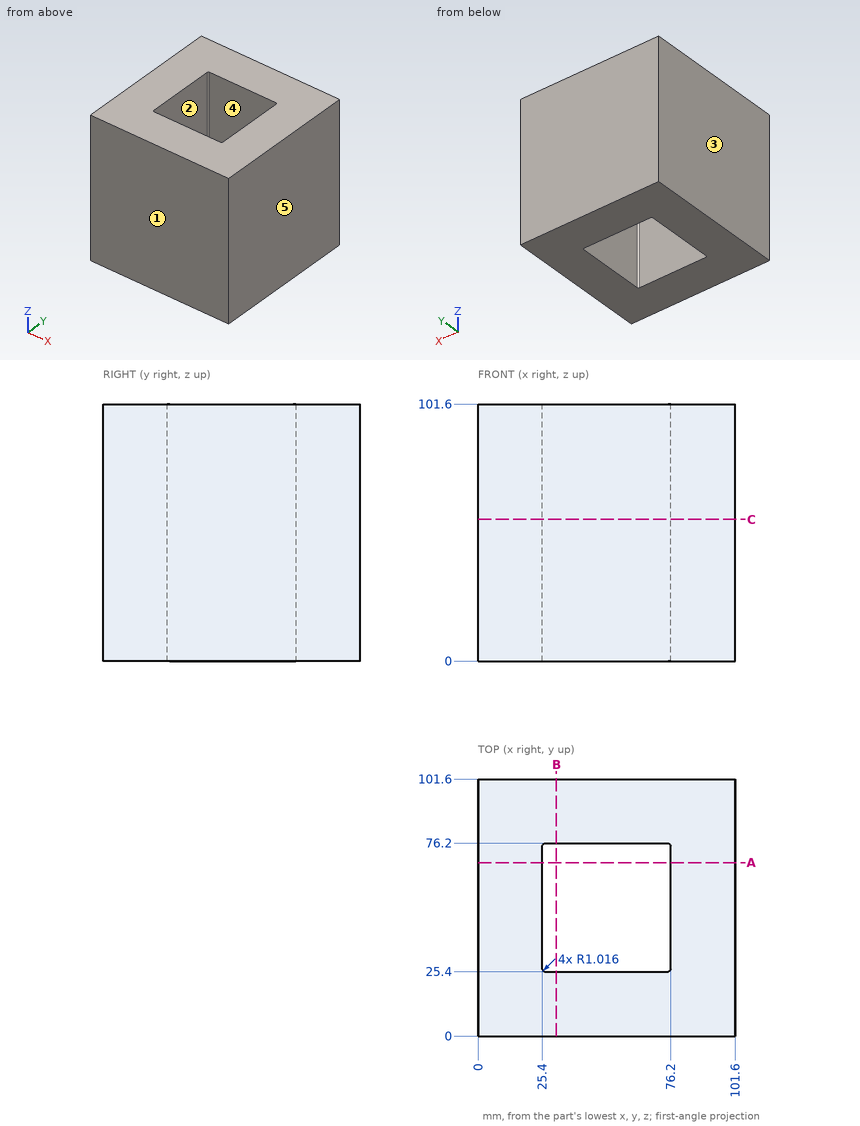
Check sheet for the drawn part. Datum: minimum x, y, z corner. Units: mm. A direction names the side the tool comes from. Round coordinates to 2 decimals unless told otherwise and drop trailing zeros. Loops run counter-clockwise (first coordinate to the right, second up) from the corner with the lowest first, then second, coordinate; pieces in that order, holes last. Notation, with made-up numbers: (5.25, 7.25) -> (43.25, 7.25) arc R22 ccw to (43.25, 18.25) -> close; hole circle Ø7 at (-5, 77.25). An arc over 180 degrees is marked (long way). Put each result on its own line as item: value. Start each with the question number.
1. Draft check along X on the marked faces 1, 2 and 3. Enter one of: +X half, -X half, draft (parallel to the pull), parting line (faces both ways), or undercut.
2. Section check C-C (z = 56). Enter the section's corners in (x, y).
3. Scan line: probe 1 along X at (y, z) = (71.5, 36). Record every from-to range of solid material in increasing order.
4. Section check A-A (y = 68.5). Enter the section's corners in (x, z), plus the area to 3 significant figures.
5. Access from +Z, -Z, +X, -X, +Y, -Y to the whole of each face (thin tool, end or side, straight path). Record for the marked faces 4 and 5.
Findings:
1. face 1: draft
1. face 2: undercut
1. face 3: -X half
2. outline: (0, 0) -> (101.6, 0) -> (101.6, 101.6) -> (0, 101.6) -> close; hole (25.4, 26.42) arc R1.02 ccw to (26.42, 25.4) -> (75.18, 25.4) arc R1.02 ccw to (76.2, 26.42) -> (76.2, 75.18) arc R1.02 ccw to (75.18, 76.2) -> (26.42, 76.2) arc R1.02 ccw to (25.4, 75.18) -> close
3. probe 1: x = 0 to 25.4, 76.2 to 101.6
4. outline: (0, 0) -> (25.4, 0) -> (25.4, 101.6) -> (0, 101.6) -> close; (76.2, 0) -> (101.6, 0) -> (101.6, 101.6) -> (76.2, 101.6) -> close
4. area: 5,160 mm^2
5. face 4: +Z, -Z
5. face 5: +Z, -Z, +X, +Y, -Y
